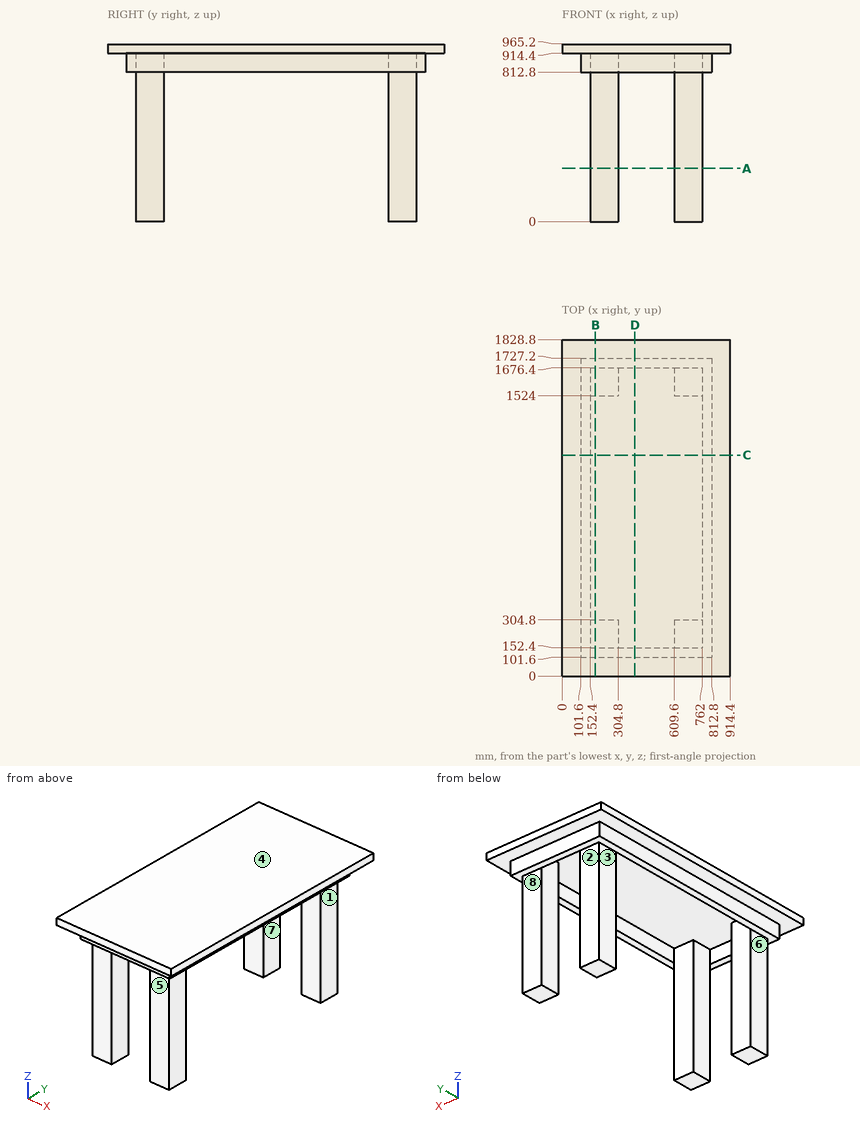
Verification items for this drawing (mm, ordinates from the low corner). A direction names the side the tool comes from. Give positions to 0.01 mm unless a question says otherwise; leave off trailing zeros. Loops run counter-clockwise (first coordinate to the right, second up) from the corner with the lowest first, then second, coordinate; pieces in that order, holes last. Notation, with made-up numbers: (31.5, 46.5) - (35.5, 46.5) arc R26 ccw to (35.5, 73.5) - close; hole circle Ø3 at (89, -20). An arc over 180 degrees is marked (long way). Write item = value, one per line. Start each with the question number.
Q1. Cross-section at C-C, the plane y = 1200. Enter the section's corners in (x, z).
Q2. Mould release check, pull along X, two halves, no side actions. Record for the marked faces 6, 7 and 8: released by +X, released by -X, zero draft, split by the parting line, or undercut.
Q3. Cross-section at B-B, the plane x = 181. Enter the section's corners in (y, z), and give its area (3 significant figures).
Q4. Depth check by flat-ended pin: P1, Ø6, axis at y = 202, z = 642, coming from the -X side; P2, Ø2, axis at x = 481.5, y = 778, coming from the -Z side. Enter the tip coordinate at first touch or a pass-through.
Q5. Cross-section at D-D, the plane x = 395.5. Enter the section's corners in (y, z).
Q6. Cross-section at A-A, the plane z = 289. Enter the section's corners in (x, y).
Q7. Thickness scan on line 1 (Y direction, x = 164, z = 853); line 2 (Y direction, x = 303, z = 496); line 3 (X direction, y = 1529.5, z = 156.5). Record the ranges inside material, lowest first.
Q8. Tool access check on the marked faces 1, 2, 3, 4 and 5. Record the directions out of +Z, -Z, +X, -X, +Y, -Y that give a thin tool (end or side, any length) a straight path to the whole face; none if there is none.
Answer key:
q1.outline = (0, 914.4) - (101.6, 914.4) - (101.6, 812.8) - (152.4, 812.8) - (152.4, 914.4) - (762, 914.4) - (762, 812.8) - (812.8, 812.8) - (812.8, 914.4) - (914.4, 914.4) - (914.4, 965.2) - (0, 965.2) - close
q2.face_6 = released by -X
q2.face_7 = undercut
q2.face_8 = zero draft
q3.outline = (0, 914.4) - (101.6, 914.4) - (101.6, 812.8) - (152.4, 812.8) - (152.4, 0) - (304.8, 0) - (304.8, 914.4) - (1524, 914.4) - (1524, 0) - (1676.4, 0) - (1676.4, 812.8) - (1727.2, 812.8) - (1727.2, 914.4) - (1828.8, 914.4) - (1828.8, 965.2) - (0, 965.2) - close
q3.area = 382,000 mm^2
q4.P1 = 152.4
q4.P2 = 914.4
q5.outline = (0, 914.4) - (101.6, 914.4) - (101.6, 812.8) - (152.4, 812.8) - (152.4, 914.4) - (1676.4, 914.4) - (1676.4, 812.8) - (1727.2, 812.8) - (1727.2, 914.4) - (1828.8, 914.4) - (1828.8, 965.2) - (0, 965.2) - close
q6.outline = (152.4, 152.4) - (304.8, 152.4) - (304.8, 304.8) - (152.4, 304.8) - close; (152.4, 1524) - (304.8, 1524) - (304.8, 1676.4) - (152.4, 1676.4) - close; (609.6, 152.4) - (762, 152.4) - (762, 304.8) - (609.6, 304.8) - close; (609.6, 1524) - (762, 1524) - (762, 1676.4) - (609.6, 1676.4) - close
q7.line_1 = 101.6 to 304.8, 1524 to 1727.2
q7.line_2 = 152.4 to 304.8, 1524 to 1676.4
q7.line_3 = 152.4 to 304.8, 609.6 to 762
q8.face_1 = -Z, +X, +Y, -Y
q8.face_2 = -Z, +X, -X, +Y
q8.face_3 = -Z, -X, +Y, -Y
q8.face_4 = +Z, +X, -X, +Y, -Y
q8.face_5 = -Z, +X, -X, -Y
